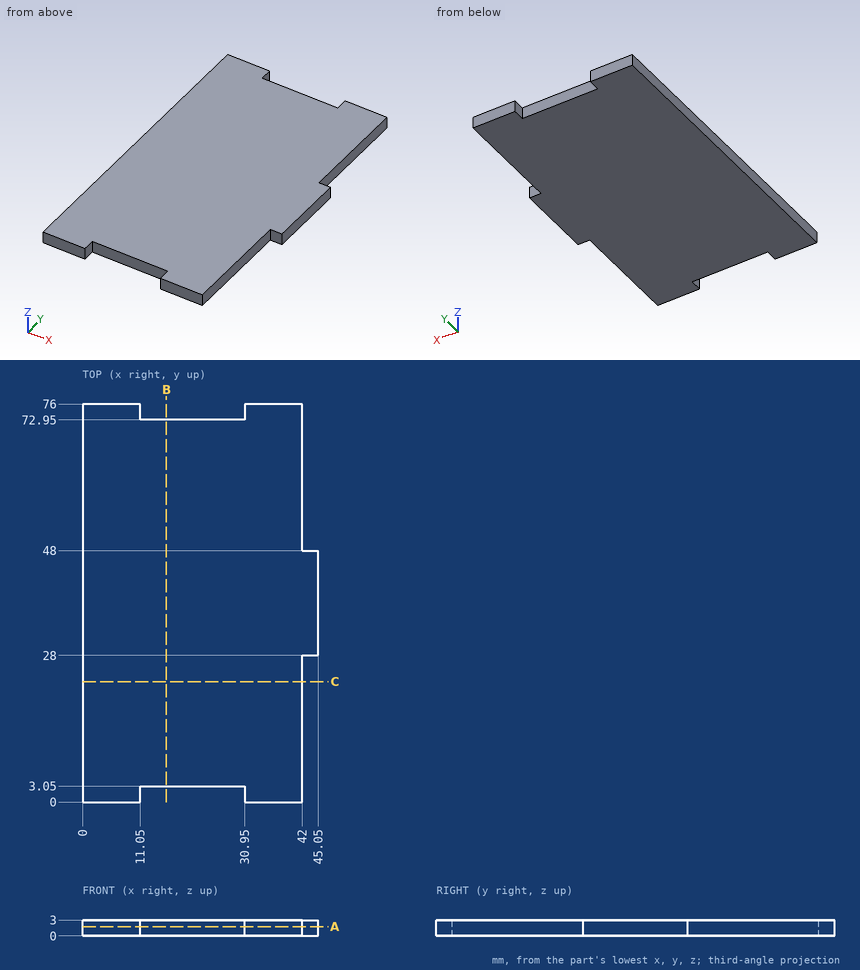
Can you work these out from the drawing? Everything is in mm from the part's minimum corner. Round coordinates to 2 decimals unless told otherwise and drop trailing zeros. Loops run counter-clockwise (first coordinate to the right, second up) from the corner with the lowest first, then second, coordinate; pieces in that order, holes last. Notation, with made-up numbers: (-0.5, 57.25) -> (31.5, 57.25) arc R33 ccw to (31.5, 96.25) -> close; hole circle Ø1 at (61.25, 78.5). An arc over 180 degrees is marked (long way). Put each result on its own line as item: value.
Q1. For pin 1 Ø0.9 at (y, z) = (1, 1) entering from +X; pin 2 Ø1.5 at (y, z) = (2, 1.5) entering from -X; pin 3 Ø1.5 at (x, z) = (44.5, 1.5) entering from +Y; pin 4 Ø1.5 at (x, z) = (25, 1.5) entering from -Y, each with a flat end and sliding along its axis, tell me the tip position at first contact or that it passes through.
Checks:
pin 1: x = 42
pin 2: x = 0
pin 3: y = 48
pin 4: y = 3.05
Q2. I want a section at A-A on z = 1.75. Write out the boundary of the cut face in (x, y), and give its area (3 significant figures).
Checks:
outline: (0, 0) -> (11.05, 0) -> (11.05, 3.05) -> (30.95, 3.05) -> (30.95, 0) -> (42, 0) -> (42, 28) -> (45.05, 28) -> (45.05, 48) -> (42, 48) -> (42, 76) -> (30.95, 76) -> (30.95, 72.95) -> (11.05, 72.95) -> (11.05, 76) -> (0, 76) -> close
area: 3,130 mm2
Q3. Please list where these lines run through material, in increasing order: line 1 (X direction, y = 27, z = 2.45); line 2 (Y direction, x = 21, z = 0.35). Write a range as from..to.
Checks:
line 1: 0..42
line 2: 3.05..72.95
Q4. I want a section at B-B on x = 16. Write out the boundary of the cut face in (y, z).
Checks:
outline: (3.05, 0) -> (72.95, 0) -> (72.95, 3) -> (3.05, 3) -> close
Q5. I want a section at C-C on y = 23. Write out the boundary of the cut face in (x, z), and give its area (3 significant figures).
Checks:
outline: (0, 0) -> (42, 0) -> (42, 3) -> (0, 3) -> close
area: 126 mm2
